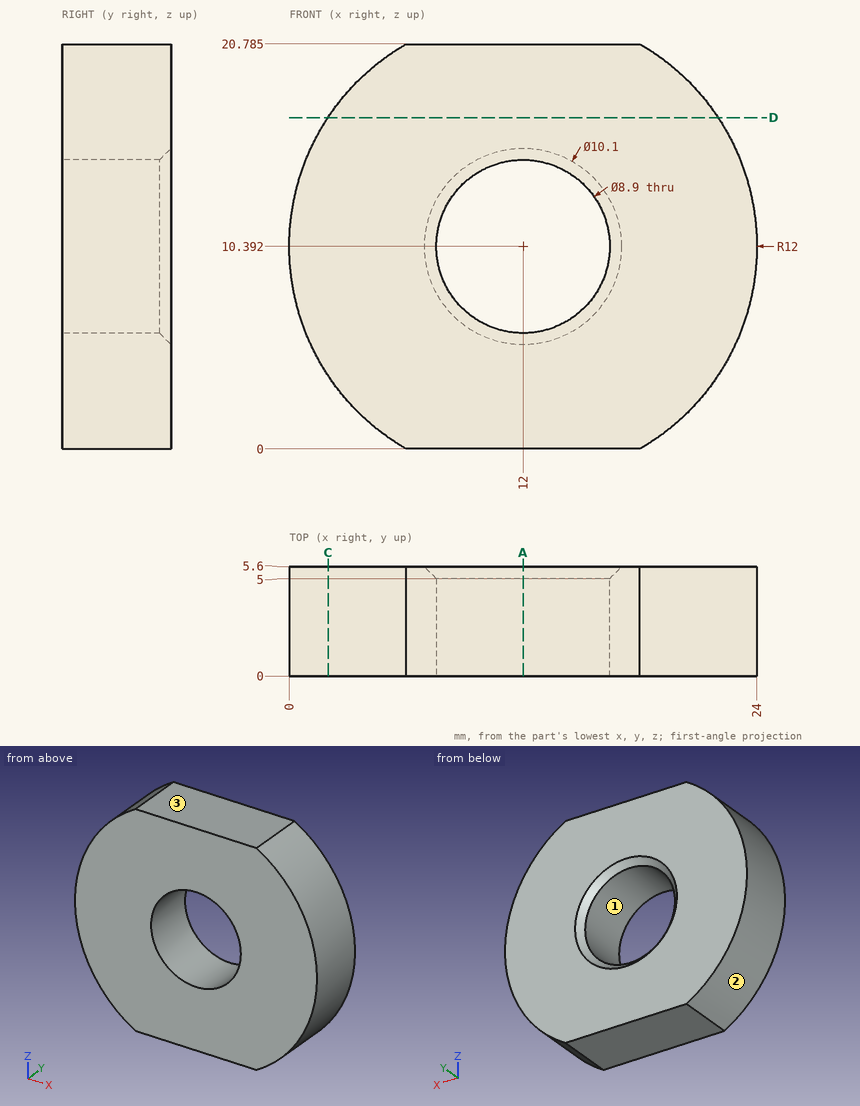
Geometry: see drawing. Coordinates: mm, zero at the bounding-box minimum. Coordinates: 2 decimals unless noted, no trailing zeros. Order: outer loops, then holes, each group sorted by start corner. A loop starts at its lowest first (then second) coordinate and runs counter-clockwise, first axis right, second up. Notation, with made-up numbers: (-34.75, 7) - (-1.75, 7) arc R19 cw to (-1.75, 19) - close; hole circle Ø2 at (-28, 83). An arc over 180 degrees is marked (long way). Return JSON: item names as keys, results as strings.
Q1. Cut plane D-D (z = 17). Return loops of the section in (x, y), then the cut area to 3 significant figures.
The answers:
{"outline": "(1.98, 0) - (22.02, 0) - (22.02, 5.6) - (1.98, 5.6) - close", "area": "112 mm2"}
Q2. Draft query along X for the marked faces 1, 2 and 3. Return one class per face: +X half, -X half, draft (parallel to the pull), parting line (faces both ways), or undercut.
The answers:
{"face 1": "undercut", "face 2": "-X half", "face 3": "draft"}
Q3. Cut plane C-C (x = 2). Return loops of the section in (y, z) (1 decimal).
The answers:
{"outline": "(0, 3.8) - (5.6, 3.8) - (5.6, 17) - (0, 17) - close"}
Q4. Ray query, probe 1 along Z at (x, y) = (12, 1.1) (1 decimal); probe 2 along Z at (x, y) = (16, 4.45) (1 decimal); probe 3 along X at (y, z) = (5.35, 9.5) (1 decimal). Return the intervals inside material, ascending.
The answers:
{"probe 1": "z = 0 to 5.9, 14.8 to 20.8", "probe 2": "z = 0 to 8.4, 12.3 to 20.8", "probe 3": "x = 0 to 7.3, 16.7 to 24"}
Q5. Cut plane A-A (x = 12). Return loops of the section in (y, z) (1 decimal).
The answers:
{"outline": "(0, 0) - (5.6, 0) - (5.6, 5.3) - (5, 5.9) - (0, 5.9) - close; (0, 14.8) - (5, 14.8) - (5.6, 15.4) - (5.6, 20.8) - (0, 20.8) - close"}
Q6. First-contact query: pin 1 (11.5 mm diameter, centred on x = 12, z = 10.39, fed in from +Y); pin 2 (1 mm diameter, centred on y = 1, z = 12, fed in from -X); pin 3 (1 mm diameter, centred on y = 1, z = 5, fed in from -X); pin 4 (3 mm diameter, centred on x = 21, y = 5, fed in from +Z). Flat tips, straight axial feed; report the tip coordinate or a pass-through.
The answers:
{"pin 1": "stops at y = 5.6", "pin 2": "stops at x = 0.05", "pin 3": "stops at x = 1.04", "pin 4": "stops at z = 19.76"}
